Here's how the part is built. I have some questions about the finished solid (model axes, mm). Round coordinates to 2 decimals unless told otherwise and drop trailing zeros. Write each loop counter-clockwise with the first axis right and the second up, starting at its lowest first coordinate (ties: lowest second). Pieces come first, ordered by that corner, then holes. Notation, with made-up numbers: (64.25, 59) - (101.25, 59) arc R11 ccw to (101.25, 66) - close; hole circle Ø9 at (36, 66). An arc over 180 degrees is marked (long way). One line per item, written item: value. Start each with the question number.
Item 1: Imagine slicing it at B-B, the plane y = 1.3. Count the separate pieces of the cut face and the enclosed holes in it, then the cut area to 3 significant figures.
Item 2: Imagine slicing it at A-A, the plane x = -13. Please give me the cut outline in (y, z), then the cut area to 3 significant figures.
Item 3: If I drill on line 1 (X direction, y = 1.65, z = -12.5), over which ranges is the centre line in solid material (lowest first)?
Item 4: For P1, Ø3.5, axis at x = -150, z = 90, coming from the -Y side, with a flat end and sliding along its axis, tell me the tip position at first contact or that it passes through.
```python
from build123d import *

# Parameters (mm, degrees)
SKETCH1_W           = 400
SKETCH1_H           = 400
BOSS_EXTRUDE1_DEPTH = 2
SKETCH2_R           = 3
CUT_EXTRUDE1_DEPTH  = 283.849783454
SKETCH3_W           = 40
SKETCH3_H           = 40
CUT_EXTRUDE2_DEPTH  = 283.849783454


with BuildPart() as part:
    # Sketch1 → Boss-Extrude1 (new body)
    with BuildSketch(Plane(origin=(0, 0, 0), x_dir=(1, 0, 0), z_dir=(0, 1, 0))):
        Rectangle(SKETCH1_W, SKETCH1_H)
    extrude(amount=BOSS_EXTRUDE1_DEPTH)

    # Sketch2 → Cut-Extrude1 (cut, through all)
    with BuildSketch(Plane(origin=(0, 2, 0), x_dir=(1, 0, 0), z_dir=(0, 1, 0))):
        with Locations(Location((-150, 150, 0), (0, 0, 270))):
            Circle(SKETCH2_R)
        with Locations(Location((-90, 150, 0), (0, 0, 270))):
            Circle(SKETCH2_R)
        with Locations(Location((-30, 150, 0), (0, 0, 270))):
            Circle(SKETCH2_R)
        with Locations(Location((30, 150, 0), (0, 0, 270))):
            Circle(SKETCH2_R)
        with Locations(Location((90, 150, 0), (0, 0, 270))):
            Circle(SKETCH2_R)
        with Locations(Location((150, 150, 0), (0, 0, 270))):
            Circle(SKETCH2_R)
        with Locations(Location((-90, 90, 0), (0, 0, 270))):
            Circle(SKETCH2_R)
        with Locations(Location((-30, 90, 0), (0, 0, 270))):
            Circle(SKETCH2_R)
        with Locations(Location((30, 90, 0), (0, 0, 270))):
            Circle(SKETCH2_R)
        with Locations(Location((90, 90, 0), (0, 0, 270))):
            Circle(SKETCH2_R)
        with Locations(Location((150, 90, 0), (0, 0, 270))):
            Circle(SKETCH2_R)
        with Locations(Location((-90, 30, 0), (0, 0, 270))):
            Circle(SKETCH2_R)
        with Locations(Location((-30, 30, 0), (0, 0, 270))):
            Circle(SKETCH2_R)
        with Locations(Location((30, 30, 0), (0, 0, 270))):
            Circle(SKETCH2_R)
        with Locations(Location((90, 30, 0), (0, 0, 270))):
            Circle(SKETCH2_R)
        with Locations(Location((150, 30, 0), (0, 0, 270))):
            Circle(SKETCH2_R)
        with Locations(Location((-90, -30, 0), (0, 0, 270))):
            Circle(SKETCH2_R)
        with Locations(Location((-30, -30, 0), (0, 0, 270))):
            Circle(SKETCH2_R)
        with Locations(Location((30, -30, 0), (0, 0, 270))):
            Circle(SKETCH2_R)
        with Locations(Location((90, -30, 0), (0, 0, 270))):
            Circle(SKETCH2_R)
        with Locations(Location((150, -30, 0), (0, 0, 270))):
            Circle(SKETCH2_R)
        with Locations(Location((-90, -90, 0), (0, 0, 270))):
            Circle(SKETCH2_R)
        with Locations(Location((-30, -90, 0), (0, 0, 270))):
            Circle(SKETCH2_R)
        with Locations(Location((30, -90, 0), (0, 0, 270))):
            Circle(SKETCH2_R)
        with Locations(Location((90, -90, 0), (0, 0, 270))):
            Circle(SKETCH2_R)
        with Locations(Location((150, -90, 0), (0, 0, 270))):
            Circle(SKETCH2_R)
        with Locations(Location((-90, -150, 0), (0, 0, 270))):
            Circle(SKETCH2_R)
        with Locations(Location((-30, -150, 0), (0, 0, 270))):
            Circle(SKETCH2_R)
        with Locations(Location((30, -150, 0), (0, 0, 270))):
            Circle(SKETCH2_R)
        with Locations(Location((90, -150, 0), (0, 0, 270))):
            Circle(SKETCH2_R)
        with Locations(Location((150, -150, 0), (0, 0, 270))):
            Circle(SKETCH2_R)
        with Locations(Location((-150, 90, 0), (0, 0, 270))):
            Circle(SKETCH2_R)
        with Locations(Location((-150, 30, 0), (0, 0, 270))):
            Circle(SKETCH2_R)
        with Locations(Location((-150, -30, 0), (0, 0, 270))):
            Circle(SKETCH2_R)
        with Locations(Location((-150, -90, 0), (0, 0, 270))):
            Circle(SKETCH2_R)
        with Locations(Location((-150, -150, 0), (0, 0, 270))):
            Circle(SKETCH2_R)
    extrude(amount=-CUT_EXTRUDE1_DEPTH, mode=Mode.SUBTRACT)

    # Sketch3 → Cut-Extrude2 (cut, through all)
    with BuildSketch(Plane(origin=(0, 2, 0), x_dir=(1, 0, 0), z_dir=(0, 1, 0))):
        Rectangle(SKETCH3_W, SKETCH3_H)
    extrude(amount=-CUT_EXTRUDE2_DEPTH, mode=Mode.SUBTRACT)


solid = part.part
```
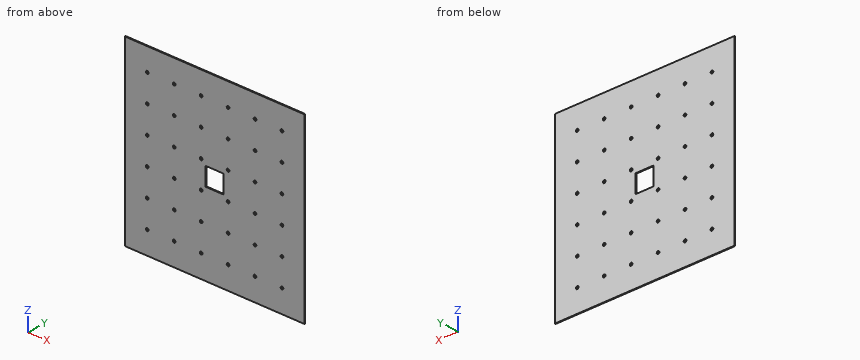
Values follow:
1. separate pieces: 1
1. enclosed holes: 37
1. area: 157,000 mm^2
2. outline: (0, -200) - (2, -200) - (2, -20) - (0, -20) - close; (0, 20) - (2, 20) - (2, 200) - (0, 200) - close
2. area: 720 mm^2
3. line 1: x = -200 to -20, 20 to 200
4. P1: passes through
